Could you check a few things on this model? Use its own coordinates, in mm. A direction names the side the tool comes from. Coordinates: 2 decimals unless noted, no trailing zeros. Order: outer loops, then holes, each group sorted by start corner. A loop starts at its lowest first (then second) coordinate and runs counter-clockwise, first axis right, second up. Notation, with made-up numbers: (-12, 17) -> (28, 17) arc R33 ccw to (28, 47) -> close; hole circle Ø5 at (77.25, -5). An arc over 180 degrees is marked (long way). Use a Markdown table: item, result. Add a question column.
1) If I drill on L1, parallel to X at y = 29, z = 0; L2, parallel to X at y = -103.5, z = -29.5; L3, parallel to Z at x = 2, y = 36.5, over which ranges is the centre line in solid material (lowest first)? Write a range as [from, to].
2) Will these pins go through, and if not, where does the flat tip stop? pin 1 Ø2 at (x, z) = (21, 28.5) entering from -Y; pin 2 Ø3 at (x, z) = (-0.5, -1.5) entering from +Y; pin 3 Ø1 at (x, z) = (-22.5, -19) entering from +Y; pin 4 Ø1.3 at (y, z) = (74.95, 0) entering from +X.
3) Which directions (+Z, -Z, +X, -X, +Y, -Y) give clear straight access to the entire face, cutting with the end or side of a thin tool? Please do faces 4 (the flat face through (-11.176, 2, 35)), 5 (the flat face through (34.2, -34.728, 5.1)), 6 (the flat face through (11.684, 2, 34)), 7 (the flat face through (-29, 127, -20)).
4) If we section it at B-B (x = 31): Give the number of separate pieces and of enclosed holes in the cut face, plus the area to 3 significant figures.
5) Thinking about a two-plate mould opening in X: for faces 1 (the flat face through (-11.176, 2, -35)), 2 (the flat face through (-13, -9.239, 34)), 3 (the flat face through (-13, -34.7, -33)), which applies, +X half, -X half, draft (parallel to the pull), parting line (faces both ways), or undercut?
6) If we section it at A-A (y = 60): Write out the boundary of the cut face in (x, z), plus the area to 3 significant figures.
```python
from build123d import *

# Parameters (mm, degrees)
F0_R     = 38.320105
F1_DEPTH = 127
F2_R     = 30
F3_T     = -4
F4_R     = 1.067549
F5_DEPTH = 50
F4_R_2   = 1.060399
F6_DEPTH = 50
F7_W     = 14.223997
F7_H     = 20.320001
F8_DEPTH = 50
F7_W_2   = 20.294623
F7_H_2   = 25.249181
F7_W_3   = 20.192685
F7_H_3   = 25.460336
F9_DEPTH = 50


with BuildPart() as f1:
    # F0 (on Front) → F1 (new body, symmetric)
    with BuildSketch(Plane.XZ):
        Circle(F0_R)
    extrude(amount=F1_DEPTH, both=True)

    # F2
    f2_edges = [f1.edges().sort_by_distance(p)[0] for p in [
        (-38.320105, -127, 0),
    ]]
    fillet(f2_edges, radius=F2_R)

    # F3
    f3_openings = [f1.faces().sort_by_distance(p)[0] for p in [
        (0, 127, 0),
    ]]
    offset(amount=F3_T, openings=f3_openings)

    # F4 (on Right) → F5 (cut, symmetric)
    with BuildSketch(Plane.YZ):
        with Locations((-75.115211, 0)):
            Circle(F4_R)
    extrude(amount=F5_DEPTH, both=True, mode=Mode.SUBTRACT)

    # F4 (on Right) → F6 (cut, symmetric)
    with BuildSketch(Plane.YZ):
        with Locations((74.953705, 0)):
            Circle(F4_R_2)
    extrude(amount=F6_DEPTH, both=True, mode=Mode.SUBTRACT)

    # F7 (on Top) → F8 (cut, symmetric)
    with BuildSketch(Plane.XY):
        with Locations((18.796, 2.285999)):
            Rectangle(F7_W, F7_H)
        with Locations((-18.288002, 2.285999)):
            Rectangle(F7_W, F7_H)
    extrude(amount=F8_DEPTH, both=True, mode=Mode.SUBTRACT)

    # F7 (on Top) → F9 (cut, symmetric)
    with BuildSketch(Plane.XY):
        with Locations((24.450503, -22.103406)):
            Rectangle(F7_W_2, F7_H_2)
        with Locations((-12.618189, -21.969469)):
            Rectangle(F7_W_3, F7_H_3)
    extrude(amount=F9_DEPTH, both=True, mode=Mode.SUBTRACT)


solid = f1.part
```
Answer sheet:
| question | item | result |
|---|---|---|
| 1 | L1 | [-38.32, -34.32], [34.32, 38.32] |
| 1 | L2 | [-23.33, -15.86], [15.86, 23.33] |
| 1 | L3 | [-38.27, -34.26], [34.26, 38.27] |
| 2 | pin 1 | y = -111.82 |
| 2 | pin 2 | y = -123 |
| 2 | pin 3 | y = -111.43 |
| 2 | pin 4 | through |
| 3 | face 4 | +Z, -Z, -X |
| 3 | face 5 | +Z, -Z |
| 3 | face 6 | +Z, -Z, +X |
| 3 | face 7 | +Z, -Z, +X, -X, +Y |
| 4 | separate pieces | 3 |
| 4 | enclosed holes | 0 |
| 4 | area | 3,500 mm2 |
| 5 | face 1 | -X half |
| 5 | face 2 | undercut |
| 5 | face 3 | draft |
| 6 | outline | circle Ø76.64 at (0, 0); hole circle Ø68.64 at (0, 0) |
| 6 | area | 913 mm2 |
